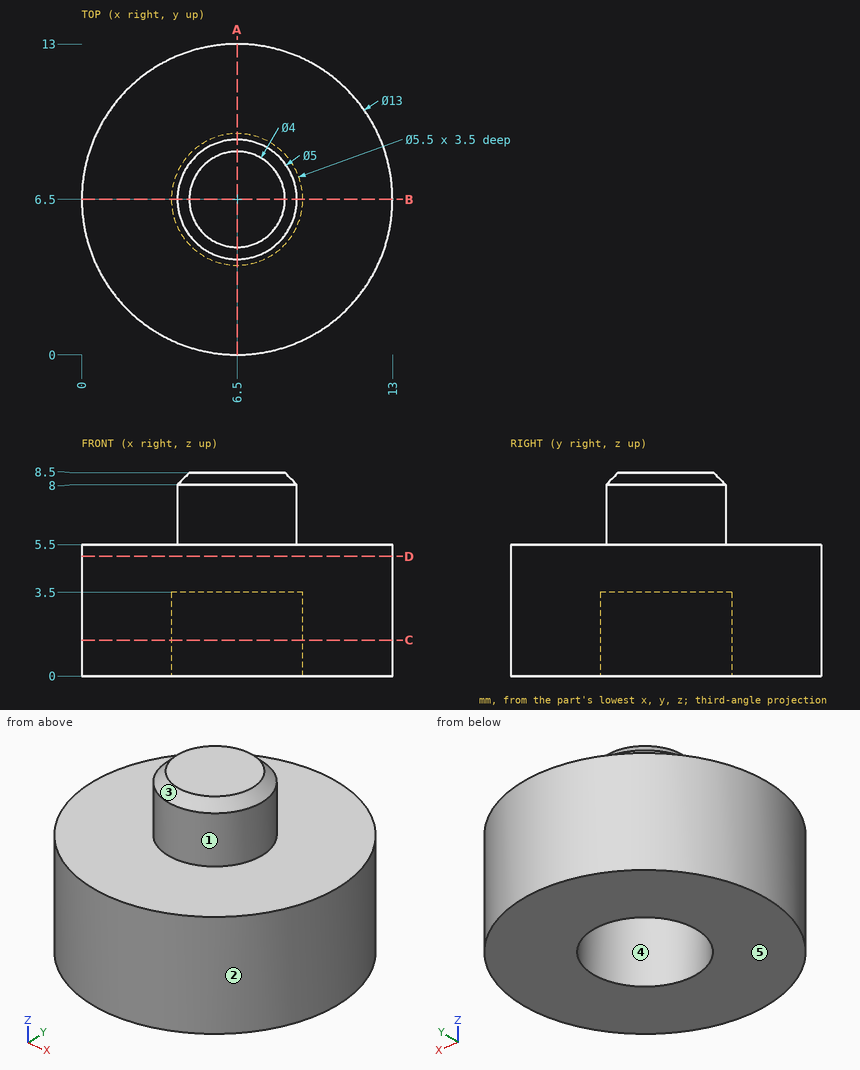
For this review, use the dimensioned drawing (mm, ordinates from the lowest corner) and the shaded views. A direction names the side the tool comes from. Give positions to 0.01 mm unless a question says otherwise; leave off trailing zeros. Order: outer loops, then holes, each group sorted by start corner. A loop starts at its lowest first (then second) coordinate and runs counter-clockwise, first axis right, second up. Notation, with made-up numbers: (60, 45.5) - (81, 45.5) arc R22 cw to (81, 62.5) - close; hole circle Ø5 at (-1, -20). An arc over 180 degrees is marked (long way). Use a Markdown table: item, result. Add a question column.
(1) Clearance check with flat-ended pins moving along their axes: P1, Ø4, axis at y = 3, z = 1, coming from the +X side; P2, Ø2, axis at y = 10, z = 3.5, coming from the +X side; P3, Ø1.6, axis at x = 7.5, y = 7, coming from the -Z side. State where each tip first meets the part, or that it passes through.
(2) Add section A-A on x = 6.5. Give the boundary of the cut face in (y, z).
(3) Machinability: for the marked faces 1 and 2, which of the approach directions +Z, -Z, +X, -X, +Y, -Y give a long, thin tool a straight path to every point of the face, cutting with its end or side? Answer none if there is none.
(4) Add section C-C on z = 1.5. Give the boundary of the cut face in (x, y), then the cut area to 3 significant figures.
(5) Wall thickness on probe 1 along Y at (x, z) = (6.5, 1.65); probe 2 along Z at (x, y) = (9, 3.5); probe 3 along X at (y, z) = (12.5, 1.5): over which ranges is each line inside the solid? List them lowest first. Write a range as [from, to].
(6) Mouldability with a two-part tool opening along Y and no side actions: class the marked faces 3, 4 and 5 as +Y half, -Y half, draft (parallel to the pull), parting line (faces both ways), or undercut.
(7) Add section D-D on z = 5. Give the boundary of the cut face in (x, y), then the cut area to 3 significant figures.
Report:
| question | item | result |
|---|---|---|
| 1 | P1 | stops at x = 12.82 |
| 1 | P2 | stops at x = 12.5 |
| 1 | P3 | stops at z = 3.5 |
| 2 | outline | (0, 0) - (3.75, 0) - (3.75, 3.5) - (9.25, 3.5) - (9.25, 0) - (13, 0) - (13, 5.5) - (9, 5.5) - (9, 8) - (8.5, 8.5) - (4.5, 8.5) - (4, 8) - (4, 5.5) - (0, 5.5) - close |
| 3 | face 1 | +Z |
| 3 | face 2 | +Z, -Z |
| 4 | outline | circle Ø13 at (6.5, 6.5); hole circle Ø5.5 at (6.5, 6.5) |
| 4 | area | 109 mm² |
| 5 | probe 1 | y = [0, 3.75], [9.25, 13] |
| 5 | probe 2 | z = [0, 5.5] |
| 5 | probe 3 | x = [4, 9] |
| 6 | face 3 | parting line |
| 6 | face 4 | undercut |
| 6 | face 5 | draft |
| 7 | outline | circle Ø13 at (6.5, 6.5) |
| 7 | area | 133 mm² |
